For this review, take the finished solid that the model builds, in its own axes (mm). A direction names the side the tool comes from. Give positions to 0.01 mm unless a question says otherwise; leave off trailing zeros. Write each loop counter-clockwise with the first axis right and the second up, starting at its lowest first coordinate (ties: lowest second). Pieces come first, ordered by that corner, then holes. Notation, with made-up numbers: (86.25, -5) -> (98.25, -5) arc R12 cw to (98.25, 16) -> close; hole circle Ø2 at (56.25, 59.25). An arc over 180 degrees is marked (long way). Return JSON: item names as keys, results as strings.
from build123d import *

# Parameters (mm, degrees)
F0_W     = 30
F0_H     = 15
F1_DEPTH = 3
F2_W     = 10
F2_H     = 8
F3_DEPTH = 8
F4_R     = 3.99999
F5_R     = 1.5
F6_DEPTH = 25
F7_R     = 1
F8_R     = 2.5
F9_DEPTH = 3
F10_R    = 0.2


# Not quite as in the source:
# - a fillet or chamfer is up to 0.001 mm smaller than in the source, because OpenCascade refuses the exact size


with BuildPart() as f1:
    # F0 (on Top) → F1 (new body)
    with BuildSketch(Plane.XY):
        with Locations((-8.5063918959, 3.0821188468)):
            Rectangle(F0_W, F0_H)
    extrude(amount=F1_DEPTH)

    # F2 (on face) → F3 (join)
    with BuildSketch(Plane.XY.offset(3)):
        with Locations((-8.5063918959, 3.0821188468)):
            Rectangle(F2_W, F2_H)
    extrude(amount=F3_DEPTH)

    # F4 (radius 4 in the source; OpenCascade refuses exactly that, so slightly less here)
    f4_edges = [f1.edges().sort_by_distance(p)[0] for p in [
        (-8.506392, -0.917881, 11),
        (-8.506392, 7.082119, 11),
    ]]
    fillet(f4_edges, radius=F4_R)

    # F5 (on face) → F6 (cut)
    with BuildSketch(Plane.YZ.offset(-3.5063918959)):
        with Locations((3.0821188468, 7)):
            Circle(F5_R)
    extrude(amount=-F6_DEPTH, mode=Mode.SUBTRACT)

    # F7
    f7_edges = [f1.edges().sort_by_distance(p)[0] for p in [
        (-23.506392, 3.082119, 3),
        (-8.506392, 10.582119, 3),
        (6.493608, 3.082119, 3),
        (-8.506392, -4.417881, 3),
    ]]
    fillet(f7_edges, radius=F7_R)

    # F8 (on face) → F9 (join)
    with BuildSketch(Plane(origin=(0, 0, 0), x_dir=(1, 0, 0), z_dir=(0, 0, -1))):
        with Locations((-16.0063918959, -3.0821188468)):
            Circle(F8_R)
        with Locations((-1.0063918959, -3.0821188468)):
            Circle(F8_R)
    extrude(amount=F9_DEPTH)

    # F10
    f10_edges = [f1.edges().sort_by_distance(p)[0] for p in [
        (-18.506392, 3.082119, -3),
        (-3.506392, 3.082119, -3),
    ]]
    fillet(f10_edges, radius=F10_R)


solid = f1.part
1. Add section B-B, the plane y = 7.75. State the section outline as (x, z) points, plus the area to 3 significant figures.
Results found:
{"outline": "(-23.51, 0) -> (6.49, 0) -> (6.49, 2) arc R1 ccw to (5.49, 3) -> (-22.51, 3) arc R1 ccw to (-23.51, 2) -> close", "area": "89.6 mm²"}
2. Add section A-A, the plane x = 4.75. State the section outline as (y, z) points.
Results found:
{"outline": "(-4.42, 0) -> (10.58, 0) -> (10.58, 2) arc R1 ccw to (9.58, 3) -> (-3.42, 3) arc R1 ccw to (-4.42, 2) -> close"}
3. The part is to be moulded in two halves that separate along X. For faces 1 (the flat face through (-8.7, -1.2, 3)), 2 (the flat face through (-9, 3, 0)), 3 (the flat face through (-13.506, 3, 5)), say which applies: +X half, -X half, draft (parallel to the pull), parting line (faces both ways), or undercut.
Results found:
{"face 1": "draft", "face 2": "undercut", "face 3": "-X half"}
4. For faces 4 (the flat face through (-9, -0.918, 5)), 5 (the flat face through (-3.506, 3, 5)), 6 (the cylindrical face through (-13.622, 2.331, -1.38)), 7 (the flat face through (-23.506, 3, 1)), 8 (the flat face through (-9, 7.082, 5)), list the 3-axis set-ups (+Z, -Z, +X, -X, +Y, -Y) from which the entire face can be reached by the end or side of a thin tool; tool diameter is ignored.
Results found:
{"face 4": "+Z, +X, -X, -Y", "face 5": "+Z, +X, +Y, -Y", "face 6": "-Z", "face 7": "+Z, -Z, -X, +Y, -Y", "face 8": "+Z, +X, -X, +Y"}
5. To check wall thickness, follow probe 1 along Z at (x, y) = (-8.75, -1.5); probe 2 along X at (y, z) = (3.5, 5.25); probe 3 along Y at (x, z) = (-7.5, 7.5). State the ranges of each line that lie inside material, in increasing order.
Results found:
{"probe 1": "z = 0 to 3", "probe 2": "x = -13.51 to -3.51", "probe 3": "y = -0.89 to 1.67, 4.5 to 7.05"}
6. For pin 1 (2 mm diameter, centred on x = -8.5, z = 4.5, fed in from -Y); pin 2 (3.5 mm diameter, centred on y = 3.08, z = 7, fed in from -X); pin 3 (6.5 mm diameter, centred on y = 4, z = 7, fed in from +X), all flat-tipped, find the tip position at first contact; note any pin that passes through.
Results found:
{"pin 1": "stops at y = -0.92", "pin 2": "stops at x = -13.51", "pin 3": "stops at x = -3.51"}
